```python
from build123d import *

# Parameters (mm, degrees)
SKETCH1_W           = 17.805
SKETCH1_H           = 20
SKETCH1_W_2         = 38
SKETCH1_H_2         = 5
BOSS_EXTRUDE1_DEPTH = 3
SKETCH3_R           = 1.5
CUT_EXTRUDE1_DEPTH  = 5
SKETCH7_W           = 15.61
SKETCH7_H           = 10
BOSS_EXTRUDE4_DEPTH = 30
BOSS_EXTRUDE5_DEPTH = 15.61
SKETCH9_R           = 1.5
CUT_EXTRUDE2_DEPTH  = 5
BOSS_EXTRUDE6_DEPTH = 8
FILLET4_R           = 2
BOSS_EXTRUDE7_DEPTH = 82


with BuildPart() as part:
    # Sketch1 → Boss-Extrude1 (new body)
    with BuildSketch(Plane(origin=(0, 0, 0), x_dir=(1, 0, 0), z_dir=(0, 1, 0))):
        Polygon((9.368218391, 0.25), (-8.436781609, 0.25), (-26.241781609, 0.25), (-38.436781609, 0.25), (-38.436781609, -4.75), (21.563218391, -4.75), (21.563218391, 0.25), align=None)
        with Locations((0.465718391, 10.25)):
            Rectangle(SKETCH1_W, SKETCH1_H)
        with Locations((-17.339281609, 10.25)):
            Rectangle(SKETCH1_W, SKETCH1_H)
        with Locations((-57.436781609, -2.25)):
            Rectangle(SKETCH1_W_2, SKETCH1_H_2)
    extrude(amount=BOSS_EXTRUDE1_DEPTH)

    # Sketch3 → Cut-Extrude1 (cut)
    with BuildSketch(Plane.XZ):
        with Locations(Location((-20.484687418, -8.75, 0), (0, 0, 270))):
            Circle(SKETCH3_R)
        with Locations(Location((-8.434877213, -16.25, 0), (0, 0, 270))):
            Circle(SKETCH3_R)
        with Locations(Location((3.614932992, -8.75, 0), (0, 0, 270))):
            Circle(SKETCH3_R)
    extrude(amount=-CUT_EXTRUDE1_DEPTH, mode=Mode.SUBTRACT)

    # Sketch7 → Boss-Extrude4 (add)
    with BuildSketch(Plane(origin=(0, 3, 0), x_dir=(1, 0, 0), z_dir=(0, 1, 0))):
        with Locations((-8.436781609, 5.25)):
            Rectangle(SKETCH7_W, SKETCH7_H)
    extrude(amount=BOSS_EXTRUDE4_DEPTH)

    # Sketch8 → Boss-Extrude5 (add)
    with BuildSketch(Plane.ZY.offset(16.241781609)):
        Polygon((-10.25, 33), (-0.25, 50.320508076), (-0.25, 33), align=None)
    extrude(amount=-BOSS_EXTRUDE5_DEPTH)

    # Sketch9 → Cut-Extrude2 (cut)
    with BuildSketch(Plane(origin=(0, 12.688380194, -21.976919162), x_dir=(1, 0, 0), z_dir=(0, 0.4999999999999978, -0.8660254037844399))):
        with Locations(Location((-11.436781609, -33.453838325, 0), (0, 0, 270))):
            Circle(SKETCH9_R)
        with Locations(Location((-5.436781609, -33.453838325, 0), (0, 0, 270))):
            Circle(SKETCH9_R)
    extrude(amount=-CUT_EXTRUDE2_DEPTH, mode=Mode.SUBTRACT)

    # Sketch2 → Boss-Extrude6 (add)
    with BuildSketch(Plane(origin=(21.563218391, 0, 0), x_dir=(0, 0, -1), z_dir=(1, 0, 0))):
        with BuildLine():
            Line((-37.762183827, 48.301156639), (-38.630424716, 43.377117874))
            ThreePointArc((-38.630424716, 43.377117874), (-14.342177832, 29.354291997), (-4.75, 3))
            Line((-4.75, 3), (0.25, 3))
            ThreePointArc((0.25, 3), (-10.511955617, 32.568230046), (-37.762183827, 48.301156639))
        make_face()
    boss_extrude6 = extrude(amount=-BOSS_EXTRUDE6_DEPTH)

    # Mirror1: Boss-Extrude6 across plane
    add(boss_extrude6.mirror(Plane.ZY.offset(27.436781609)))

    # Fillet4
    fillet4_edges = [part.edges().sort_by_distance(p)[0] for p in [
        (-76.436781609, 29.354291997, 14.342177832),
        (-76.436781609, 32.568230046, 10.511955617),
        (-76.436781609, 45.839137256, 38.196304271),
        (21.563218391, 0, 2.25),
        (21.563218391, 1.5, 4.75),
        (21.563218391, 1.5, -0.25),
        (-76.436781609, 1.5, -0.25),
        (-76.436781609, 1.5, 4.75),
        (-76.436781609, 0, 2.25),
        (21.563218391, 29.354291997, 14.342177832),
        (-27.436781609, 0, 4.75),
        (21.563218391, 32.568230046, 10.511955617),
        (21.563218391, 45.839137256, 38.196304271),
    ]]
    fillet(fillet4_edges, radius=FILLET4_R)

    # Sketch10 → Boss-Extrude7 (add)
    with BuildSketch(Plane(origin=(-68.436781609, 0, 0), x_dir=(0, 0, -1), z_dir=(1, 0, 0))):
        with BuildLine():
            ThreePointArc((-32.079730178, 41.653896608), (-31.378929062, 41.398858318), (-30.682882682, 41.131115585))
            ThreePointArc((-30.682882682, 41.131115585), (-29.29976717, 41.733383141), (-28.730833488, 43.130540682))
            ThreePointArc((-28.730833488, 43.130540682), (-31.537743217, 44.960539777), (-32.079730178, 41.653896608))
        make_face()
    extrude(amount=BOSS_EXTRUDE7_DEPTH)


solid = part.part
```
Build history of the part. All positions in model axes, mm. A direction names the side the tool comes from. Round coordinates to 2 decimals unless told otherwise and drop trailing zeros. Write each loop counter-clockwise with the first axis right and the second up, starting at its lowest first coordinate (ties: lowest second). Pieces come first, ordered by that corner, then holes.
1) Band-saw the part on D-D, the plane y = 21.5. Give the number of separate pieces and of enclosed holes in the cut face, and give its area (3 significant figures).
2) Pin check, flat tips, straight feed: pin 1 (3.5 mm diameter, centred on y = 1.5, z = -7, fed in from -X); pin 2 (2.5 mm diameter, centred on x = 14, y = 1, fed in from -Z); pin 3 (6 mm diameter, centred on y = 25.5, z = -5.5, fed in from -X). Stop position of each tip, or through.
3) Drill centre lines: probe 1 along X at (y, z) = (0.8, -8.75); probe 2 along X at (y, z) = (0.95, -16.25); probe 3 along Z at (x, y) = (-11, 13). Where is each one in solid material? Low to high.
4) Band-saw the part on B-B, the plane z = -16.25. List the corners of the cut face in (x, y).
5) Band-saw the part on C-C, the plane z = -8.75. List the corners of the cut face in (x, y), and give its area (3 significant figures).
6) Band-saw the part on A-A, the plane x = -27.5. List the corners of the cut face in (y, z), and give its area (3 significant figures).
7) Mould opens along Z. For faces 1 (the cylindrical face through (3.68, 1.48, -7.25)), 2 (the flat face through (15, 1, -0.25)), 3 (the flat face through (-16.242, 22, -5)) say: +Z half, -Z half, draft (parallel to the pull), parting line (faces both ways), or undercut.
8) 3-axis set-ups, long thin cutter, end or side, ignore diameter. For faces 4 (the flat face through (9.368, 1, -10)), 5 (the flat face through (-50, 1, -0.25)), 6 (the flat face through (-9, 18, -10.25)), 7 (the cylindrical face through (20.96, 2.51, 4.18)): which of +Z, -Z, +X, -X, +Y, -Y reach the whole face in a straight line?
Ans:
1. separate pieces: 3
1. enclosed holes: 0
1. area: 241 mm2
2. pin 1: stops at x = -26.24
2. pin 2: stops at z = -0.25
2. pin 3: stops at x = -16.24
3. probe 1: x = -26.24 to -21.98, -18.98 to 2.11, 5.11 to 9.37
3. probe 2: x = -26.24 to -9.93, -6.93 to 9.37
3. probe 3: z = -10.25 to -0.25
4. outline: (-26.24, 0) - (-9.93, 0) - (-9.93, 3) - (-26.24, 3) - close; (-6.93, 0) - (9.37, 0) - (9.37, 3) - (-6.93, 3) - close
5. outline: (-26.24, 0) - (-21.98, 0) - (-21.98, 3) - (-26.24, 3) - close; (-18.98, 0) - (2.11, 0) - (2.11, 3) - (-0.63, 3) - (-0.63, 35.6) - (-16.24, 35.6) - (-16.24, 3) - (-18.98, 3) - close; (5.11, 0) - (9.37, 0) - (9.37, 3) - (5.11, 3) - close
5. area: 598 mm2
6. outline: (0, -0.25) - (3, -0.25) - (3, 4.75) - (2, 4.75) arc R2 ccw to (0, 2.75) - close; (41.13, 30.68) arc R2 ccw (long way) to (41.65, 32.08) arc R41 cw to start
6. area: 26.6 mm2
7. face 1: undercut
7. face 2: -Z half
7. face 3: draft
8. face 4: -Z, +X, +Y, -Y
8. face 5: -Z, -X, +Y, -Y
8. face 6: -Z, +X, -X, +Y
8. face 7: +Z, +X, -Y
